```python
from build123d import *

# Parameters (mm, degrees)
SKETCH_1_R          = 5
EXTRUDE_1_DEPTH     = 3.4
SKETCH_1_3_R        = 2.55
CUT_EXTRUDE_1_DEPTH = 2.4
SKETCH_2_R          = 3.35
EXTRUDE_2_DEPTH     = 0.2
EXTRUDE_START       = 0.2
SKETCH_2_3_R        = 3.35
SKETCH_2_3_R_2      = 2.4
EXTRUDE_3_DEPTH     = 8


with BuildPart() as part:
    # 草图1 → 凸台-拉伸1 (new body)
    with BuildSketch(Plane(origin=(0, 0, 0), x_dir=(1, 0, 0), z_dir=(0, 1, 0))):
        with Locations(Location((0, 0, 0), (0, 0, 270))):
            Circle(SKETCH_1_R)
    extrude(amount=EXTRUDE_1_DEPTH)

    # 草图1<3> → 切除-拉伸1 (cut)
    with BuildSketch(Plane(origin=(0, 0, 0), x_dir=(1, 0, 0), z_dir=(0, 1, 0))):
        with Locations(Location((0, 0, 0), (0, 0, 270))):
            Circle(SKETCH_1_3_R)
    extrude(amount=CUT_EXTRUDE_1_DEPTH, mode=Mode.SUBTRACT)

    # 草图2 → 凸台-拉伸2 (add)
    with BuildSketch(Plane(origin=(0, 3.4, 0), x_dir=(1, 0, 0), z_dir=(0, 1, 0))):
        with Locations(Location((0, 0, 0), (0, 0, 270))):
            Circle(SKETCH_2_R)
    extrude(amount=EXTRUDE_2_DEPTH)

    # 草图2<3> → 凸台-拉伸3 (add)
    # profile 1 of 5: a face of its own
    with BuildSketch(Plane(origin=(0, 3.4, 0), x_dir=(1, 0, 0), z_dir=(0, 1, 0)).offset(EXTRUDE_START)):
        with Locations(Location((0, 0, 0), (0, 0, 270))):
            Circle(SKETCH_2_3_R)
        Circle(SKETCH_2_3_R_2, mode=Mode.SUBTRACT)
    # profile 2 of 5: a face of its own
    with BuildSketch(Plane(origin=(0, 3.4, 0), x_dir=(1, 0, 0), z_dir=(0, 1, 0)).offset(EXTRUDE_START)):
        with BuildLine():
            Line((-1.121727474, 1.121727474), (-1.121727474, 2.121727474))
            ThreePointArc((-1.121727474, 2.121727474), (-1.697056275, 1.697056275), (-2.121727474, 1.121727474))
            Line((-2.121727474, 1.121727474), (-1.121727474, 1.121727474))
        make_face()
    # profile 3 of 5: a face of its own
    with BuildSketch(Plane(origin=(0, 3.4, 0), x_dir=(1, 0, 0), z_dir=(0, 1, 0)).offset(EXTRUDE_START)):
        with BuildLine():
            ThreePointArc((2.121727474, 1.121727474), (1.697056275, 1.697056275), (1.121727474, 2.121727474))
            Line((1.121727474, 2.121727474), (1.121727474, 1.121727474))
            Line((1.121727474, 1.121727474), (2.121727474, 1.121727474))
        make_face()
    # profile 4 of 5: a face of its own
    with BuildSketch(Plane(origin=(0, 3.4, 0), x_dir=(1, 0, 0), z_dir=(0, 1, 0)).offset(EXTRUDE_START)):
        with BuildLine():
            Line((-1.121727474, -2.121727474), (-1.121727474, -1.121727474))
            Line((-1.121727474, -1.121727474), (-2.121727474, -1.121727474))
            ThreePointArc((-2.121727474, -1.121727474), (-1.697056275, -1.697056275), (-1.121727474, -2.121727474))
        make_face()
    # profile 5 of 5: a face of its own
    with BuildSketch(Plane(origin=(0, 3.4, 0), x_dir=(1, 0, 0), z_dir=(0, 1, 0)).offset(EXTRUDE_START)):
        with BuildLine():
            Line((2.121727474, -1.121727474), (1.121727474, -1.121727474))
            Line((1.121727474, -1.121727474), (1.121727474, -2.121727474))
            ThreePointArc((1.121727474, -2.121727474), (1.697056275, -1.697056275), (2.121727474, -1.121727474))
        make_face()
    extrude(amount=EXTRUDE_3_DEPTH)


solid = part.part
```
Here's how the part is built. I have some questions about the finished solid (model axes, mm). A direction names the side the tool comes from. Round coordinates to 2 decimals unless told otherwise and drop trailing zeros. Loops run counter-clockwise (first coordinate to the right, second up) from the corner with the lowest first, then second, coordinate; pieces in that order, holes last. Notation, with made-up numbers: (78, 35.5) -> (136, 35.5) arc R18 ccw to (136, 66.5) -> close; hole circle Ø9 at (52, 46). An arc over 180 degrees is marked (long way). Answer as CSV lines item,"result".
1. Thinking about a two-plate mould opening in X: for faces 4 (the face through (-3.3, 3.4, -1.2)), 5 (the face through (0, 3.6, 0)), 6 (the face through (-2.038, 7.443, -2.658)), which applies, released by +X, released by -X, zero draft, split by the parting line, or undercut?
Final values:
face 4,"zero draft"
face 5,"undercut"
face 6,"split by the parting line"
2. Which directions (+Z, -Z, +X, -X, +Y, -Y) give clear straight access to the entire face, cutting with the end or side of a thin tool? Please do faces 1 (the face through (-4.88, 1.68, -1.08)), 2 (the face through (-1.6, 7.5, 1.122)), 3 (the face through (0, 2.4, 0)).
Final values:
face 1,"+Y, -Y"
face 2,"+Y"
face 3,"-Y"
3. If I drill on L1, parallel to X at y = 1.55, z = 0; L2, parallel to X at y = 9.75, z = 0.25; L3, parallel to Y at x = 0.5, z = -2.25, over which ranges is the centre line in solid material (lowest first)?
Final values:
L1,"x = -5 to -2.55, 2.55 to 5"
L2,"x = -3.34 to -2.39, 2.39 to 3.34"
L3,"y = 2.4 to 3.6"
4. If we section it at A-A on y = 6.5: Please give me the cut outline in (x, z).
Final values:
outline,"circle Ø6.7 at (0, 0); hole (-2.12, -1.12) -> (-1.12, -1.12) -> (-1.12, -2.12) arc R2.4 ccw to (1.12, -2.12) -> (1.12, -1.12) -> (2.12, -1.12) arc R2.4 ccw to (2.12, 1.12) -> (1.12, 1.12) -> (1.12, 2.12) arc R2.4 ccw to (-1.12, 2.12) -> (-1.12, 1.12) -> (-2.12, 1.12) arc R2.4 ccw to start"
5. If we section it at D-D on y = 3: Please give me the cut outline in (x, z).
Final values:
outline,"circle Ø10 at (0, 0)"
6. If we section it at B-B on z = 0: Please give me the cut outline in (x, y).
Final values:
outline,"(-5, 0) -> (-2.55, 0) -> (-2.55, 2.4) -> (2.55, 2.4) -> (2.55, 0) -> (5, 0) -> (5, 3.4) -> (3.35, 3.4) -> (3.35, 11.6) -> (2.4, 11.6) -> (2.4, 3.6) -> (-2.4, 3.6) -> (-2.4, 11.6) -> (-3.35, 11.6) -> (-3.35, 3.4) -> (-5, 3.4) -> close"
7. For pin 1 (1.5 mm diameter, centred on x = 2, y = 6, fed in from -Z); pin 2 (1.1 mm diameter, centred on y = 9, z = -1.5, fed in from -X); pin 3 (1 mm diameter, centred on x = -2.5, y = 4.5, fed in from +Z), each with a flat end and sliding along its axis, tell me the tip position at first contact or that it passes through.
Final values:
pin 1,"stops at z = -3.11"
pin 2,"stops at x = -3.21"
pin 3,"stops at z = 2.69"
8. If we section it at C-C on x = 0: Please give me the cut outline in (y, z), plus the area to 3 significant figures.
Final values:
outline,"(0, -5) -> (3.4, -5) -> (3.4, -3.35) -> (11.6, -3.35) -> (11.6, -2.4) -> (3.6, -2.4) -> (3.6, 2.4) -> (11.6, 2.4) -> (11.6, 3.35) -> (3.4, 3.35) -> (3.4, 5) -> (0, 5) -> (0, 2.55) -> (2.4, 2.55) -> (2.4, -2.55) -> (0, -2.55) -> close"
area,"38.3 mm^2"
